For this review, take the finished solid that the model builds, in its own axes (mm). A direction names the side the tool comes from. Round coordinates to 2 decimals unless told otherwise and drop trailing zeros. Loops run counter-clockwise (first coordinate to the right, second up) from the corner with the lowest first, then second, coordinate; pieces in that order, holes last. Notation, with made-up numbers: (85, 43.25) -> (126, 43.25) arc R14 cw to (126, 47.25) -> close; hole circle Ø6 at (29, 73.25). An arc over 180 degrees is marked (long way). Write each question's results on one line, items separated by ' | '.
```python
from build123d import *

# Parameters (mm, degrees)
SKETCH1_W               = 400
SKETCH1_H               = 400
SKETCH1_W_2             = 396
SKETCH1_H_2             = 396
BOSS_EXTRUDE1_DEPTH     = 300
CUT_LOFT1_START         = 2
CUT_LOFT1_DEPTH         = 396
BOSS_EXTRUDE2_DEPTH     = 400
BOSS_EXTRUDE3_DEPTH     = 2
BOSS_EXTRUDE6_START     = -398
BOSS_EXTRUDE6_DEPTH     = 2
CUT_EXTRUDE1_DEPTH      = 641.312423915
CUT_EXTRUDE1_DEPTH_BACK = 641.312423915
SKETCH9_R               = 6
BOSS_EXTRUDE4_START     = -2
SKETCH10_R              = 16
SKETCH10_R_2            = 14
BOSS_EXTRUDE4_DEPTH     = 16
BOSS_EXTRUDE5_START     = -18
SKETCH11_R              = 16
SKETCH11_R_2            = 14
BOSS_EXTRUDE5_DEPTH     = 16
CUT_EXTRUDE2_DEPTH      = 720.739536394
CUT_EXTRUDE2_DEPTH_BACK = 720.739536394
SKETCH13_R              = 30
SKETCH14_R              = 3.5
BOSS_EXTRUDE7_DEPTH     = 15
BOSS_EXTRUDE8_START     = -415
SKETCH14_2_R            = 3.5
BOSS_EXTRUDE8_DEPTH     = 15


# Read off the part's stored shape, not the designer's step: Cut-Loft1
with BuildPart() as part:
    # Sketch1 → Boss-Extrude1 (new body)
    with BuildSketch(Plane(origin=(0, 0, 0), x_dir=(1, 0, 0), z_dir=(0, 1, 0))):
        with Locations((200, -200)):
            Rectangle(SKETCH1_W, SKETCH1_H)
        with Locations((200, -200)):
            Rectangle(SKETCH1_W_2, SKETCH1_H_2, mode=Mode.SUBTRACT)
    extrude(amount=BOSS_EXTRUDE1_DEPTH)

    # Upper_profile → Loft6 section 0
    with BuildSketch(Plane(origin=(0, 0, 0), x_dir=(1, 0, 0), z_dir=(0, 1, 0))):
        with BuildLine():
            Line((0, 0), (400, 0))
            Line((400, 0), (400, -400))
            Line((400, -400), (0, -400))
            Line((0, -400), (0, 0))
        make_face()
    # Bellow_profile → Loft6 section 1
    with BuildSketch(Plane(origin=(0, -100, 0), x_dir=(1, 0, 0), z_dir=(0, 1, 0))):
        with BuildLine():
            Line((155, 0), (245, 0))
            Line((245, 0), (245, -400))
            Line((245, -400), (155, -400))
            Line((155, -400), (155, 0))
        make_face()
    loft()

    # Cut-Loft1 outline → Cut-Loft1 (cut)
    with BuildSketch(Plane.XY.offset(CUT_LOFT1_START)):
        Polygon((157, -100), (243, -100), (398, 0), (2, 0), align=None)
    extrude(amount=CUT_LOFT1_DEPTH, mode=Mode.SUBTRACT)

    # Sketch7 → Boss-Extrude2 (add)
    with BuildSketch(Plane.XY.offset(400)):
        with BuildLine():
            Line((155, -100), (157, -100))
            ThreePointArc((157, -100), (200, -143), (243, -100))
            Line((243, -100), (245, -100))
            ThreePointArc((245, -100), (200, -145), (155, -100))
        make_face()
    extrude(amount=-BOSS_EXTRUDE2_DEPTH)

    # Sketch8 → Boss-Extrude3 (add)
    with BuildSketch(Plane.XY.offset(400)):
        with BuildLine():
            Line((245, -100), (155, -100))
            ThreePointArc((155, -100), (200, -145), (245, -100))
        make_face()
    extrude(amount=-BOSS_EXTRUDE3_DEPTH)

    # Sketch8<2> → Boss-Extrude6 (add)
    with BuildSketch(Plane.XY.offset(400).offset(BOSS_EXTRUDE6_START)):
        with BuildLine():
            Line((245, -100), (155, -100))
            ThreePointArc((155, -100), (200, -145), (245, -100))
        make_face()
    extrude(amount=-BOSS_EXTRUDE6_DEPTH)

    # Sketch9 → Cut-Extrude1 (cut, two sides: drawn at the far end of the back side and taken through both)
    with BuildSketch(Plane.XY.offset(400).offset(-CUT_EXTRUDE1_DEPTH_BACK)):
        with Locations(Location((200, -100, 0), (0, 0, 180))):
            Circle(SKETCH9_R)
    extrude(amount=CUT_EXTRUDE1_DEPTH + CUT_EXTRUDE1_DEPTH_BACK, mode=Mode.SUBTRACT)

    # Sketch10 → Boss-Extrude4 (add)
    with BuildSketch(Plane.XY.offset(400).offset(BOSS_EXTRUDE4_START)):
        with Locations(Location((200, -100, 0), (0, 0, 180))):
            Circle(SKETCH10_R)
        with Locations(Location((200, -100, 0), (0, 0, 180))):
            Circle(SKETCH10_R_2, mode=Mode.SUBTRACT)
    extrude(amount=-BOSS_EXTRUDE4_DEPTH)

    # Sketch11 → Boss-Extrude5 (add)
    with BuildSketch(Plane(origin=(0, 0, 0), x_dir=(-1, 0, 0), z_dir=(0, 0, -1)).offset(BOSS_EXTRUDE5_START)):
        with Locations((-200, -100)):
            Circle(SKETCH11_R)
        with Locations((-200, -100)):
            Circle(SKETCH11_R_2, mode=Mode.SUBTRACT)
    extrude(amount=BOSS_EXTRUDE5_DEPTH)

    # Sketch13 → Cut-Extrude2 (cut, two sides: drawn at the far end of the back side and taken through both)
    with BuildSketch(Plane(origin=(0, 300, 0), x_dir=(1, 0, 0), z_dir=(0, 1, 0)).offset(-CUT_EXTRUDE2_DEPTH_BACK)):
        with Locations(Location((200, -52, 0), (0, 0, 270))):
            Circle(SKETCH13_R)
    extrude(amount=CUT_EXTRUDE2_DEPTH + CUT_EXTRUDE2_DEPTH_BACK, mode=Mode.SUBTRACT)

    # Sketch14 → Boss-Extrude7 (add)
    with BuildSketch(Plane.XY.offset(400)):
        with Locations(Location((224, -100, 0), (0, 0, 180))):
            Circle(SKETCH14_R)
        with Locations(Location((176, -100, 0), (0, 0, 180))):
            Circle(SKETCH14_R)
    extrude(amount=BOSS_EXTRUDE7_DEPTH)

    # Sketch14<2> → Boss-Extrude8 (add)
    with BuildSketch(Plane.XY.offset(400).offset(BOSS_EXTRUDE8_START)):
        with Locations(Location((224, -100, 0), (0, 0, 180))):
            Circle(SKETCH14_2_R)
        with Locations(Location((176, -100, 0), (0, 0, 180))):
            Circle(SKETCH14_2_R)
    extrude(amount=BOSS_EXTRUDE8_DEPTH)


solid = part.part
```
1. Consider section A-A (y = 16). State the section outline as (x, z) points, plus the area to 3 significant figures.
Values found:
outline: (0, 0) -> (400, 0) -> (400, 400) -> (0, 400) -> close; hole (2, 2) -> (398, 2) -> (398, 398) -> (2, 398) -> close | area: 3,180 mm2
2. For pin 1 (4 mm diameter, centred on x = 264.5, y = 166, fed in from -Z); pin 2 (1 mm diameter, centred on y = -16, z = 164, fed in from -X) (3 decimals); pin 3 (12 mm diameter, centred on x = 314.5, z = 161.5, fed in from -Y); pin 4 (9.5 mm diameter, centred on x = 200, y = -100, fed in from -Z), all flat-tipped, find the tip position at first contact; note any pin that passes through.
Values found:
pin 1: stops at z = 0 | pin 2: stops at x = 24.025 | pin 3: stops at y = -59.03 | pin 4: passes through
3. Tool access review of faces 1 (the face through (200.99, -144.99, 202.8)), 2 (the face through (211.793, -110.814, 390.112)), 3 (the face through (398, 148, 203)): name each direction out of +Z, -Z, +X, -X, +Y, -Y from which nothing blocks a thin tool from reaching the whole face with its end or side.
Values found:
face 1: +Z, -Z, -Y | face 2: none | face 3: +Y
4. To check wall thickness, follow probe 1 along Y at (x, z) = (200, 392.5); probe 2 along X at (y, z) = (195, 249.5). State the ranges of each line that lie inside material, in increasing order.
Values found:
probe 1: y = -145 to -143, -116 to -114, -86 to -84 | probe 2: x = 0 to 2, 398 to 400
5. Draft analysis for pull direction Y (two halves, no side actions). For faces 4 (the face through (319.415, -50.7, 197.228)), 5 (the face through (206, -103, 2)), 6 (the face through (206, -103, 398)), 7 (the face through (2, 148, 203)), state which applies: released by +Y, released by -Y, zero draft, split by the parting line, or undercut.
Values found:
face 4: released by +Y | face 5: undercut | face 6: undercut | face 7: zero draft
6. Consider section D-D (z = 353.5). State the section outline as (x, y) points.
Values found:
outline: (0, 0) -> (155, -100) arc R45 ccw to (245, -100) -> (400, 0) -> (400, 300) -> (398, 300) -> (398, 0) -> (243, -100) arc R43 cw to (157, -100) -> (2, 0) -> (2, 300) -> (0, 300) -> close
7. Consider section B-B (z = 52). State the section outline as (x, y) points, plus the area to 3 significant figures.
Values found:
outline: (0, 0) -> (155, -100) arc R45 ccw to (170, -133.54) -> (170, -130.81) arc R43 cw to (157, -100) -> (2, 0) -> (2, 300) -> (0, 300) -> close; (230, -133.54) arc R45 ccw to (245, -100) -> (400, 0) -> (400, 300) -> (398, 300) -> (398, 0) -> (243, -100) arc R43 cw to (230, -130.81) -> close | area: 1,740 mm2
8. Consider section C-C (x = 200). Give the number of separate pieces and of enclosed holes in the cut face, plus the area to 3 significant figures.
Values found:
separate pieces: 4 | enclosed holes: 0 | area: 2,530 mm2
